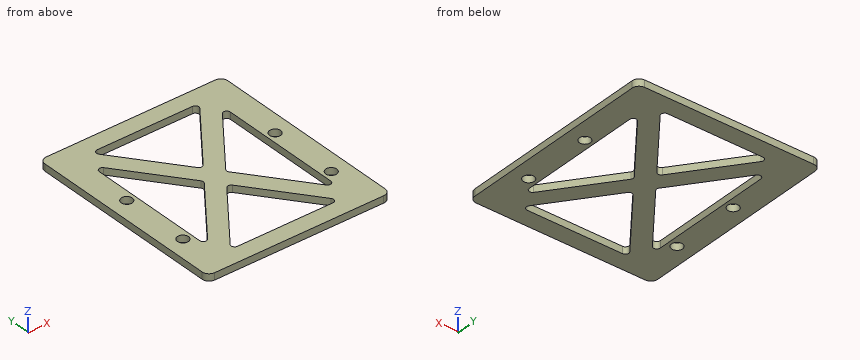
from build123d import *

# Parameters (mm, degrees)
SKETCH_1_W          = 53
SKETCH_1_H          = 60
EXTRUDE_1_DEPTH     = 2
FILLET_1_R          = 2
SKETCH_2_R          = 1.6
CUT_EXTRUDE_1_DEPTH = 41.078048855
CUT_EXTRUDE_2_DEPTH = 41.078048855
FILLET_2_R          = 1


with BuildPart() as part:
    # 草图1 → 凸台-拉伸1 (new body)
    with BuildSketch(Plane.XY):
        Rectangle(SKETCH_1_W, SKETCH_1_H)
    extrude(amount=EXTRUDE_1_DEPTH)

    # 圆角1
    fillet_1_edges = [part.edges().sort_by_distance(p)[0] for p in [
        (26.5, -30, 1),
        (-26.5, -30, 1),
        (-26.5, 30, 1),
        (26.5, 30, 1),
    ]]
    fillet(fillet_1_edges, radius=FILLET_1_R)

    # 草图2 → 切除-拉伸1 (cut, through all)
    with BuildSketch(Plane.XY.offset(2)):
        with Locations((21.5, 5)):
            Circle(SKETCH_2_R)
        with Locations((21.5, -15)):
            Circle(SKETCH_2_R)
        with Locations((-21.5, 5)):
            Circle(SKETCH_2_R)
        with Locations((-21.5, -15)):
            Circle(SKETCH_2_R)
    extrude(amount=-CUT_EXTRUDE_1_DEPTH, mode=Mode.SUBTRACT)

    # 草图3 → 切除-拉伸2 (cut, through all)
    with BuildSketch(Plane.XY.offset(2)):
        Polygon((-3.140063694, 0), (-19, 20.868337245), (-19, -20.868337245), align=None)
        Polygon((15.859936306, -25), (0, -4.131662755), (-15.859936306, -25), align=None)
        Polygon((19, 20.868337245), (3.140063694, 0), (19, -20.868337245), align=None)
        Polygon((15.859936306, 25), (-15.859936306, 25), (0, 4.131662755), align=None)
    extrude(amount=-CUT_EXTRUDE_2_DEPTH, mode=Mode.SUBTRACT)

    # 圆角2
    fillet_2_edges = [part.edges().sort_by_distance(p)[0] for p in [
        (3.140063694, 0, 1),
        (19, 20.868337245, 1),
        (19, -20.868337245, 1),
        (0, -4.131662755, 1),
        (15.859936306, -25, 1),
        (-15.859936306, -25, 1),
        (-15.859936306, 25, 1),
        (15.859936306, 25, 1),
        (0, 4.131662755, 1),
        (-19, 20.868337245, 1),
        (-3.140063694, 0, 1),
        (-19, -20.868337245, 1),
    ]]
    fillet(fillet_2_edges, radius=FILLET_2_R)


solid = part.part
Here's how the part is built. I have some questions about the finished solid (model axes, mm). Round coordinates to 2 decimals unless told otherwise and drop trailing zeros. Write each loop counter-clockwise with the first axis right and the second up, starting at its lowest first coordinate (ties: lowest second). Pieces come first, ordered by that corner, then holes. Notation, with made-up numbers: (48.25, 12.25) -> (69.25, 12.25) arc R13 cw to (69.25, 37.25) -> close; hole circle Ø11 at (20, -39). An arc over 180 degrees is marked (long way). One line per item, written item: value.
1) If I drill on line 1 (Y direction, x = 21.5, z = 1.15); line 2 (X direction, y = -10.5, z = 1.6); line 3 (Y direction, x = -7.5, z = 0.3), over which ranges is the centre line in solid material (lowest first)? Write a range as [from, to].
Filled sheet:
line 1: y = [-30, -16.6], [-13.4, 3.4], [6.6, 30]
line 2: x = [-26.5, -19], [-11.12, -4.84], [4.84, 11.12], [19, 26.5]
line 3: y = [-30, -25], [-14, -5.74], [5.74, 14], [25, 30]
2) Suppose I cut it at B-B on x = 21.5. List the corners of the cut face in (y, z) for me.
Filled sheet:
outline: (-30, 0) -> (-16.6, 0) -> (-16.6, 2) -> (-30, 2) -> close; (-13.4, 0) -> (3.4, 0) -> (3.4, 2) -> (-13.4, 2) -> close; (6.6, 0) -> (30, 0) -> (30, 2) -> (6.6, 2) -> close
3) Suppose I cut it at A-A on x = -18. List the corners of the cut face in (y, z) for me.
Filled sheet:
outline: (-30, 0) -> (-18.9, 0) -> (-18.9, 2) -> (-30, 2) -> close; (18.9, 0) -> (30, 0) -> (30, 2) -> (18.9, 2) -> close
4) Suppose I cut it at D-D on x = -12.5. List the corners of the cut face in (y, z) for me, plus the area to 3 significant figures.
Filled sheet:
outline: (-30, 0) -> (-25, 0) -> (-25, 2) -> (-30, 2) -> close; (-20.58, 0) -> (-12.32, 0) -> (-12.32, 2) -> (-20.58, 2) -> close; (12.32, 0) -> (20.58, 0) -> (20.58, 2) -> (12.32, 2) -> close; (25, 0) -> (30, 0) -> (30, 2) -> (25, 2) -> close
area: 53.1 mm2
5) I'm going to push a flat-ended pin straight in: pin 1 Ø1.9 at (x, y) = (-21.5, 5) entering from +Z. Where does the tip first touch, or does it pass through?
Filled sheet:
pin 1: passes through
6) Suppose I cut it at C-C on y = -15. List the corners of the cut face in (x, z) for me, plus the area to 3 significant figures.
Filled sheet:
outline: (-26.5, 0) -> (-23.1, 0) -> (-23.1, 2) -> (-26.5, 2) -> close; (-19.9, 0) -> (-19, 0) -> (-19, 2) -> (-19.9, 2) -> close; (-14.54, 0) -> (-8.26, 0) -> (-8.26, 2) -> (-14.54, 2) -> close; (8.26, 0) -> (14.54, 0) -> (14.54, 2) -> (8.26, 2) -> close; (19, 0) -> (19.9, 0) -> (19.9, 2) -> (19, 2) -> close; (23.1, 0) -> (26.5, 0) -> (26.5, 2) -> (23.1, 2) -> close
area: 42.3 mm2
